```python
from build123d import *

# Parameters (mm, degrees)
F1_DEPTH       = 2.25
F1_DEPTH_BACK  = 2.25
F3_DEPTH       = 20
F10_DEPTH      = 2.251
F10_DEPTH_BACK = 25


# Not quite as in the source:
# - a feature names something its author has since deleted; it is built from what else it names


with BuildPart() as f1:
    # F0 (on Top) → F1 (new body, two sides)
    with BuildSketch(Plane.XY) as f1_sk:
        Polygon((10, 50), (0, 50), (21.6506350946, 12.5), (29.1506350946, 16.8301270189), align=None)
        Polygon((-21.6506350946, 12.5), (0, 50), (-10, 50), (-29.1506350946, 16.8301270189), align=None)
        Polygon((21.6506350946, 12.5), (0, 50), (0, 0), align=None)
        Polygon((0, 0), (0, 50), (-21.6506350946, 12.5), align=None)
        Polygon((29.1506350946, 16.8301270189), (21.6506350946, 12.5), (43.3012701892, -25), (48.3012701892, -16.3397459622), align=None)
        Polygon((43.3012701892, -25), (21.6506350946, 12.5), (0, 0), align=None)
        Polygon((43.3012701892, -25), (0, 0), (-43.3012701892, -25), align=None)
        Polygon((-43.3012701892, -25), (0, 0), (-21.6506350946, 12.5), align=None)
        Polygon((-43.3012701892, -25), (-21.6506350946, 12.5), (-29.1506350946, 16.8301270189), (-48.3012701892, -16.3397459622), align=None)
        Polygon((38.3012701892, -33.6602540378), (43.3012701892, -25), (-43.3012701892, -25), (-38.3012701892, -33.6602540378), align=None)
    extrude(amount=F1_DEPTH)
    extrude(f1_sk.sketch, amount=-F1_DEPTH_BACK)


with BuildPart() as f3:
    # F2 (on face) → F3 (new body)
    with BuildSketch(Plane(origin=(0, 50, 0), x_dir=(-1, 0, 0), z_dir=(0, 1, 0))):
        with BuildLine():
            Line((-8, 0), (-6.5, 0))
            ThreePointArc((-6.5, 0), (-6.9393398282, 1.0606601718), (-8, 1.5))
            Line((-8, 1.5), (-8, 0))
        make_face()
        with BuildLine():
            ThreePointArc((-9.5, 0), (-8, -1.5), (-6.5, 0))
            Line((-6.5, 0), (-8, 0))
            Line((-8, 0), (-9.5, 0))
        make_face()
        with BuildLine():
            Line((-8, 0), (-8, 1.5))
            ThreePointArc((-8, 1.5), (-9.0606601718, 1.0606601718), (-9.5, 0))
            Line((-9.5, 0), (-8, 0))
        make_face()
    extrude(amount=-F3_DEPTH)


with BuildPart() as f3b:
    # F2 (on face) → F3, piece 2 (new body)
    with BuildSketch(Plane(origin=(0, 50, 0), x_dir=(-1, 0, 0), z_dir=(0, 1, 0))):
        with BuildLine():
            ThreePointArc((8, 1.5), (6.9393398282, 1.0606601718), (6.5, 0))
            Line((6.5, 0), (8, 0))
            Line((8, 0), (8, 1.5))
        make_face()
        with BuildLine():
            Line((8, 0), (6.5, 0))
            ThreePointArc((6.5, 0), (8, -1.5), (9.5, 0))
            Line((9.5, 0), (8, 0))
        make_face()
        with BuildLine():
            ThreePointArc((9.5, 0), (9.0606601718, 1.0606601718), (8, 1.5))
            Line((8, 1.5), (8, 0))
            Line((8, 0), (9.5, 0))
        make_face()
    extrude(amount=-F3_DEPTH)


with BuildPart() as f6_1:
    # F6: instance of F3
    add(f3.part.mirror(Plane(origin=(0, 0, 0), x_dir=(0.8660254038, 0.5, 0), z_dir=(0.5, -0.8660254038, 0))))


with BuildPart() as f6_2:
    # F6: instance of F3b
    add(f3b.part.mirror(Plane(origin=(0, 0, 0), x_dir=(0.8660254038, 0.5, 0), z_dir=(0.5, -0.8660254038, 0))))


with BuildPart() as f7_1:
    # F7: instance of F3
    add(f3.part.mirror(Plane(origin=(0, 0, 0), x_dir=(0.8660254038, -0.5, 0), z_dir=(-0.5, -0.8660254038, 0))))


with BuildPart() as f7_2:
    # F7: instance of F3b
    add(f3b.part.mirror(Plane(origin=(0, 0, 0), x_dir=(0.8660254038, -0.5, 0), z_dir=(-0.5, -0.8660254038, 0))))


with BuildPart() as f1_1:
    add(f1.part)

    # F8: cut F3, F3b, F6_1, F6_2, F7_2, F7_1
    add(f3.part, mode=Mode.SUBTRACT)
    add(f3b.part, mode=Mode.SUBTRACT)
    add(f6_1.part, mode=Mode.SUBTRACT)
    add(f6_2.part, mode=Mode.SUBTRACT)
    add(f7_2.part, mode=Mode.SUBTRACT)
    add(f7_1.part, mode=Mode.SUBTRACT)

    # F9 (on Top) → F10 (cut, two sides)
    with BuildSketch(Plane.XY) as f10_sk:
        Polygon((0, 50), (-6, 50), (0, 40), align=None)
        Polygon((0, 50), (0, 40), (6, 50), align=None)
        Polygon((-40.3012701892, -30.1961524227), (-34.6410161514, -20), (-43.3012701892, -25), align=None)
        Polygon((-43.3012701892, -25), (-34.6410161514, -20), (-46.3012701892, -19.8038475773), align=None)
        Polygon((34.6410161514, -20), (43.3012701892, -25), (46.3012701892, -19.8038475773), align=None)
        Polygon((40.3012701892, -30.1961524227), (43.3012701892, -25), (34.6410161514, -20), align=None)
    extrude(amount=-F10_DEPTH, mode=Mode.SUBTRACT)
    extrude(f10_sk.sketch, amount=F10_DEPTH_BACK, mode=Mode.SUBTRACT)


solid = f1_1.part
```
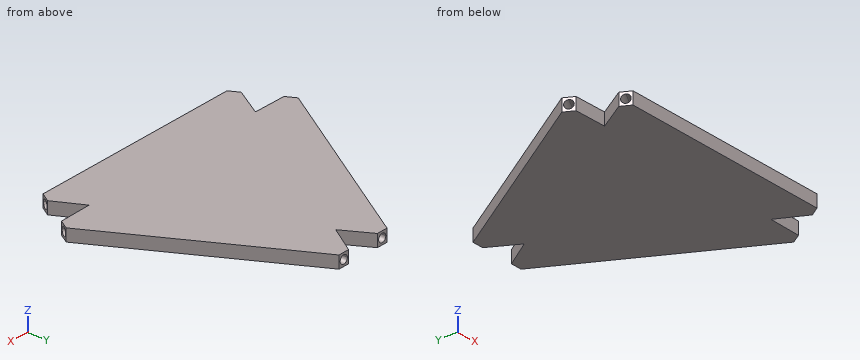
Verification items for the finished model (mm, model axes). Give positions to 0.01 mm unless a question says otherwise; leave off trailing zeros. Write each loop counter-clockwise with the first axis right and the second up, starting at its lowest first coordinate (ties: lowest second). Pieces come first, ordered by that corner, then holes. Notation, with made-up numbers: M 78.25,71 L 137.25,71 A20 ccw 137.25,94 Z; hole C -7,9 d7. An arc over 180 degrees is marked long. One line per question, with ' | ' between items.
1) Section check B-B on y = 18.5. Enter the section's corners in (x, z).
Result:
outline: M -28.19,-2.25 L 28.19,-2.25 L 28.19,2.25 L -28.19,2.25 Z
2) Thickness scan on line 1 along Y through (x, z) = (37, 0.2); line 2 along X through (y, z) = (-13, -0.25); line 3 along X through (y, z) = (-23.5, -0.2). Record the ranges inside material, lowest first. Write a range as [from, to].
Result:
line 1: y = [-33.66, -32.32], [-28.88, -24.25], [-19.96, -13.84], [-10.41, 3.23] | line 2: x = [-46.37, -41.47], [-35.56, 35.56], [41.47, 46.37] | line 3: x = [-36.58, -27.68], [-21.73, 21.73], [27.68, 36.58]
3) Section check A-A on x = -16. Enter the section's corners in (y, z), plus the area to 3 significant figures.
Result:
outline: M -33.66,-2.25 L 39.61,-2.25 L 39.61,2.25 L -33.66,2.25 Z | area: 330 mm2
4) Gauge pin test, flat ends, axial feed: pin 1 Ø1 at (y, z) = (-11, 0.5) entering from +X; pin 2 Ø0.9 at (x, z) = (8.5, 0.5) entering from +Y. Record the tip position at first contact, or that the pin passes through.
Result:
pin 1: stops at x = 45.51 | pin 2: stops at y = 30
